```python
from build123d import *

# Parameters (mm, degrees)
SKETCH1_W           = 313
SKETCH1_H           = 342
BOSS_EXTRUDE1_DEPTH = 6.35
SKETCH3_W           = 22
SKETCH3_H           = 155.14040353
SKETCH3_R           = 2.5
BOSS_EXTRUDE2_DEPTH = 6.35
SKETCH2_R           = 2.5
CUT_EXTRUDE1_DEPTH  = 7.35
SKETCH4_R           = 2.6
SKETCH4_R_2         = 2.55
CUT_EXTRUDE2_DEPTH  = 7.35


with BuildPart() as part:
    # Sketch1 → Boss-Extrude1 (new body)
    with BuildSketch(Plane(origin=(0, 0, 0), x_dir=(1, 0, 0), z_dir=(0, 1, 0))):
        Rectangle(SKETCH1_W, SKETCH1_H)
    extrude(amount=-BOSS_EXTRUDE1_DEPTH)

    # Sketch3 → Boss-Extrude2 (add)
    with BuildSketch(Plane(origin=(0, 0, 0), x_dir=(1, 0, 0), z_dir=(0, 1, 0))):
        with Locations((167.5, 9)):
            Rectangle(SKETCH3_W, SKETCH3_H)
        with Locations((166.5, 9)):
            Circle(SKETCH3_R, mode=Mode.SUBTRACT)
        with Locations((166.5, -41.8)):
            Circle(SKETCH3_R, mode=Mode.SUBTRACT)
        with Locations((166.5, 59.8)):
            Circle(SKETCH3_R, mode=Mode.SUBTRACT)
    extrude(amount=-BOSS_EXTRUDE2_DEPTH)

    # Sketch2 → Cut-Extrude1 (cut, through all)
    with BuildSketch(Plane(origin=(0, 0, 0), x_dir=(1, 0, 0), z_dir=(0, 1, 0))):
        with Locations((0, -143)):
            Circle(SKETCH2_R)
        with Locations((-70, -143)):
            Circle(SKETCH2_R)
        with Locations((70, -143)):
            Circle(SKETCH2_R)
        with Locations((-70, 161)):
            Circle(SKETCH2_R)
        with Locations((0, 161)):
            Circle(SKETCH2_R)
        with Locations((70, 161)):
            Circle(SKETCH2_R)
    extrude(amount=-CUT_EXTRUDE1_DEPTH, mode=Mode.SUBTRACT)

    # Sketch4 → Cut-Extrude2 (cut, through all)
    with BuildSketch(Plane(origin=(0, 0, 0), x_dir=(1, 0, 0), z_dir=(0, 1, 0))):
        with Locations((103.249710043, -82.783250091)):
            Circle(SKETCH4_R)
        with Locations((38.349710043, -82.783250091)):
            Circle(SKETCH4_R)
        with Locations((-51.750289957, -82.783250091)):
            Circle(SKETCH4_R)
        with Locations((-116.650289957, -82.783250091)):
            Circle(SKETCH4_R)
        with Locations((103.156346537, 71.010318364)):
            Circle(SKETCH4_R)
        with Locations((38.256346537, 71.010318364)):
            Circle(SKETCH4_R)
        with Locations((-52.687463488, 48.130966948)):
            Circle(SKETCH4_R_2)
        with Locations((-107.687463488, 48.130966948)):
            Circle(SKETCH4_R_2)
        with Locations((-52.687463488, 103.130966948)):
            Circle(SKETCH4_R_2)
        with Locations((-107.687463488, 103.130966948)):
            Circle(SKETCH4_R_2)
    extrude(amount=-CUT_EXTRUDE2_DEPTH, mode=Mode.SUBTRACT)


solid = part.part
```
Read the model definition and answer for the solid it produces. Units are mm, in the model's axes. Give positions to 0.01 mm unless a question says otherwise; leave off trailing zeros.
Item 1: The part is cut by section A-A (y = -3.25). Give the number of separate pieces and of enclosed holes in the cut face, and give its area (3 significant figures).
Item 2: This flat-tipped pin is pushed along its axis until it touches: pin 1 Ø1.9 at (x, y) = (166.5, -4.5) entering from +Z. Where does it stop, or does it pass through?
Item 3: Find the intervals of material crossed by line 1 along Z through (x, y) = (38.5, -4.5); line 2 along Z through (x, y) = (70, -2.25); line 3 along X through (y, z) = (-4.25, -9), in increasing order.
Taken from the geometry:
1. separate pieces: 1
1. enclosed holes: 19
1. area: 110,000 mm2
2. pin 1: stops at z = 68.57
3. line 1: z = -171 to -73.6, -68.42 to 80.19, 85.38 to 171
3. line 2: z = -171 to -163.5, -158.5 to 140.5, 145.5 to 171
3. line 3: x = -156.5 to 164, 169 to 178.5
